Autodesk Inventor part; units mm, degrees
ref_plane "YZ Plane" through (0, 0, 0) normal (1, 0, 0) x (0, 1, 0)
ref_plane "XZ Plane" through (0, 0, 0) normal (0, 1, 0) x (-1, 0, 0)
ref_plane "XY Plane" through (0, 0, 0) normal (0, 0, 1) x (1, 0, 0)
sketch "Sketch1" plane through (0, 0, 0) normal (0, 1, 0) x (-1, 0, 0)
  circle A0 centre (0, 0) radius 1.5
  dimension "d0" = 3
extrude "Extrusion1" add sketch "Sketch1" along normal blind 10
sketch "Sketch2" plane through (0, 10, 0) normal (0, 1, 0) x (1, 0, 0)
  line L0 (0, 0) -> (0, 4.95)
  line L1 (0, 4.95) -> (-5.95, 4.95)
  line L2 (-5.95, 4.95) -> (5.95, 4.95)
  line L3 (5.95, 4.95) -> (5.95, -4.95)
  line L4 (5.95, -4.95) -> (-5.95, -4.95)
  line L5 (-5.95, -4.95) -> (-5.95, 4.95)
  dimension "d3" = 4.95
  dimension "d4" = 5.95
  dimension "d5" = 11.9
  dimension "d6" = 9.9
extrude "Extrusion2" add sketch "Sketch2" along normal blind 9
sketch "Sketch3" plane through (0, 19, 0) normal (0, 1, 0) x (1, 0, 0)
  line L0 (0, 0) -> (6, 0)
  line L1 (6, 0) -> (6, 5)
  line L2 (6, 5) -> (-6, 5)
  line L3 (-6, 5) -> (-6, -5)
  line L4 (-6, -5) -> (6, -5)
  line L5 (6, -5) -> (6, 5)
  dimension "d9" = 6
  dimension "d10" = 5
  dimension "d11" = 12
  dimension "d12" = 10
extrude "Extrusion3" add sketch "Sketch3" along normal blind 16
properties part number "motor"
Could you check a few things on this model? Use its own coordinates, in mm. A direction names the side the tool comes from. Coordinates: 2 decimals unless noted, no trailing zeros. Loops run counter-clockwise (first coordinate to the right, second up) from the corner with the lowest first, then second, coordinate; pieces in that order, holes last.
1. Imagine slicing it at A-A (x = 0). Please give me the cut outline in (y, z).
2. Imagine slicing it at D-D (x = 5.25). Please give me the cut outline in (y, z), and give its area (3 significant figures).
3. Imagine slicing it at B-B (z = 0). Please give me the cut outline in (x, y), and give its area (3 significant figures).
4. Imagine slicing it at C-C (y = 12.5). Please give me the cut outline in (x, z).
5. For faces 1 (the face through (5.95, 14, 0)), 2 (the face through (-5.95, 14, 0)), 3 (the face through (1.2, 10, -1.2)), 4 (the face through (0, 14, -4.95)), which set-ups out of +Z, -Z, +X, -X, +Y, -Y let a thin tool reach every point of the face, with its end or its side?
6. For P1, Ø3, axis at x = -1, z = 3.5, coming from the -Y side; P2, Ø4.5, axis at y = 16.5, z = 0, coming from the +X side, each with a flat end and sliding along its axis, tell me the tip position at first contact or that it passes through.
7. I need wall thicknesses on L1, parallel to X at y = 18, z = -2.5; L2, parallel to Y at x = -3.5, z = 1; L3, parallel to Z at x = -5.5, y = 11. Which ranges of each line are inside material? Lowest first, please.
Computed values:
1. outline: (0, -1.5) - (10, -1.5) - (10, -4.95) - (19, -4.95) - (19, -5) - (35, -5) - (35, 5) - (19, 5) - (19, 4.95) - (10, 4.95) - (10, 1.5) - (0, 1.5) - close
2. outline: (10, -4.95) - (19, -4.95) - (19, -5) - (35, -5) - (35, 5) - (19, 5) - (19, 4.95) - (10, 4.95) - close
2. area: 249 mm2
3. outline: (-6, 19) - (-5.95, 19) - (-5.95, 10) - (-1.5, 10) - (-1.5, 0) - (1.5, 0) - (1.5, 10) - (5.95, 10) - (5.95, 19) - (6, 19) - (6, 35) - (-6, 35) - close
3. area: 329 mm2
4. outline: (-5.95, -4.95) - (5.95, -4.95) - (5.95, 4.95) - (-5.95, 4.95) - close
5. face 1: +Z, -Z, +X, -Y
5. face 2: +Z, -Z, -X, -Y
5. face 3: -Y
5. face 4: -Z, +X, -X, -Y
6. P1: stops at y = 10
6. P2: stops at x = 5.95
7. L1: x = -5.95 to 5.95
7. L2: y = 10 to 35
7. L3: z = -4.95 to 4.95
